The model under review builds one solid part; all positions refer to its coordinate system, in mm. Face numbers are marked on the shaded views. Round coordinates to 2 decimals unless told otherwise and drop trailing zeros. Loops run counter-clockwise (first coordinate to the right, second up) from the corner with the lowest first, then second, coordinate; pieces in that order, holes last. Notation, with made-up numbers: M 16,48.5 L 24,48.5 A18 cw 24,62.5 Z; hole C -21,-4 d4. An arc over 180 degrees is marked long. Answer in a Markdown table with one row per item. Add a question column.
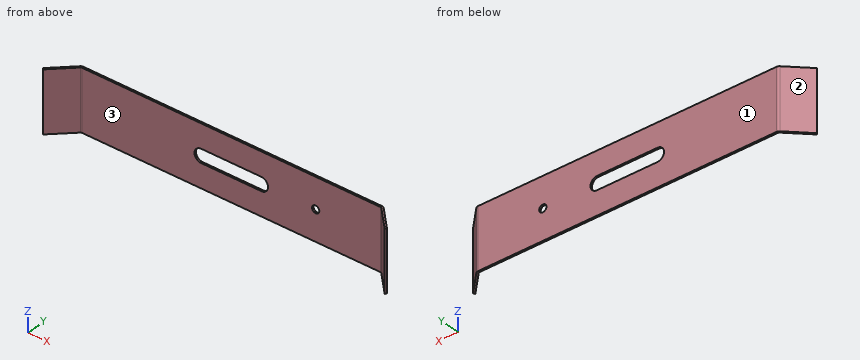
Autodesk Inventor part; units mm, degrees
ref_plane "YZ Plane" through (0, 0, 0) normal (1, 0, 0) x (0, 1, 0)
ref_plane "XZ Plane" through (0, 0, 0) normal (0, 1, 0) x (-1, 0, 0)
ref_plane "XY Plane" through (0, 0, 0) normal (0, 0, 1) x (1, 0, 0)
sketch "Sketch4" plane through (0, 0, 0) normal (0, 1, 0) x (-1, 0, 0)
  line L0 (125, 25) -> (-125, 25)
  line L1 (-125, 25) -> (-125, -25)
  line L2 (-125, -25) -> (125, -25)
  line L3 (125, -25) -> (125, 25)
  line L4 (125, 25) -> (-125, -25) construction
  line L5 (-125, 25) -> (125, -25) construction
  line L6 (25, 0) -> (-25, 0) construction
  line L7 (25, 5.5) -> (-25, 5.5)
  line L8 (-25, -5.5) -> (25, -5.5)
  arc A0 (25, -5.5) -> (25, 5.5) centre (25, 0) ccw
  arc A1 (-25, 5.5) -> (-25, -5.5) centre (-25, 0) ccw
  point P0 (0, 0)
  point P1 (0, 0)
  dimension "d17" = 250
  dimension "d18" = 50
  dimension "d19" = 50
  dimension "d20" = 11
extrude "Plate3" add sketch "Sketch4" along normal blind 1.5
sketch "Sketch6" plane through (-123.9393, 0.4393, -25) normal (-0.7071068, 0.7071068, 0) x (-0.7071068, -0.7071068, 0)
  line L0 (0, 50) -> (0, 0)
  line L1 (0, 0) -> (25, 0)
  line L2 (25, 0) -> (25, 50)
  line L3 (25, 50) -> (0, 50)
edge flange "Flange3" height 25 angle 45 thickness 1.5 bend radius 1.5 thickness toward (-0.7071068, 0.7071068, 0) relief tear relief width 1.5 relief depth 0.75 corner gap 1.5 corner form 0 edges at (-125, 0, 0) (125, 0, 0) wall of the first edge with corners at (-123.9393, 0.4393, 25) (-123.9393, 0.4393, -25) (-141.617, -17.2383, -25) (-141.617, -17.2383, 25)
bend "Bend3"
corner "Corner3"
sketch "Sketch7" plane through (0, 1.5, 0) normal (0, 1, 0) x (1, 0, 0)
  circle A0 centre (70, 0) radius 3
  point P0 (0, 0)
  dimension "d43" = 70
  dimension "d44" = 6
extrude "Cut2" cut sketch "Sketch7" against normal blind 1.5
equation "\"d41\" = Thickness"
equation "\"d2\" = Thickness"
equation "\"d31\" = BendReliefWidth"
equation "\"d32\" = BendReliefDepth"
equation "\"d33\" = MinimumRemnant"
equation "\"d34\" = TransitionRadius"
equation "\"d37\" = BendRadius"
equation "\"d38\" = CornerReliefSize"
equation "\"d39\" = GapSize"
equation "\"d40\" = JacobiRadiusSize"
equation "\"BendRadius\" = Thickness"
equation "\"BendReliefWidth\" = Thickness"
equation "\"BendReliefDepth\" = 0.5 * Thickness"
equation "\"CornerReliefSize\" = 4 * Thickness"
equation "\"MinimumRemnant\" = 2 * Thickness"
equation "\"TransitionRadius\" = BendRadius"
equation "\"JacobiRadiusSize\" = BendRadius"
equation "\"GapSize\" = Thickness"
properties part number "2309HCMUTE-CDT23_TAY-GAT" material "Stainless Steel"
1. For pin 1 Ø10 at (y, z) = (-2, 10.5) entering from -X; pin 2 Ø1 at (y, z) = (-10.5, 13) entering from -X; pin 3 Ø25 at (x, z) = (-12.5, -2.5) entering from -Y, all flat-tipped, find the tip position at first contact; note any pin that passes through.
2. Mouldability with a two-part tool opening along X and no side actions: class the marked faces 1, 2 and 3 as released by +X, released by -X, zero draft, split by the parting line, or undercut.
3. Take a section at D-D, the plane x = 41. State the section outline as (y, z) points.
4. To check wall thickness, follow probe 1 along X at (y, z) = (0.8, 0); probe 2 along X at (y, z) = (0.6, 0); probe 3 along Z at (x, y) = (70, 0.3). State the ranges of each line that lie inside material, in increasing order.
5. Take a section at C-C, the plane z = -10.5. State the section outline as (x, y) points.
6. Take a section at A-A, the plane x = 70. State the section outline as (y, z) points, and give its area (3 significant figures).
7. Take a section at B-B, the plane y = -7. State the section outline as (x, z) points, and give its area (3 significant figures).
Check sheet entries:
| question | item | result |
|---|---|---|
| 1 | pin 1 | stops at x = -133.5 |
| 1 | pin 2 | stops at x = -137.5 |
| 1 | pin 3 | stops at y = 0 |
| 2 | face 1 | zero draft |
| 2 | face 2 | released by -X |
| 2 | face 3 | undercut |
| 3 | outline | M 0,-25 L 1.5,-25 L 1.5,25 L 0,25 Z |
| 4 | probe 1 | x = -125.68 to -30.5, 30.5 to 67, 73 to 125.68 |
| 4 | probe 2 | x = -125.9 to -30.5, 30.5 to 67, 73 to 125.9 |
| 4 | probe 3 | z = -25 to -3, 3 to 25 |
| 5 | outline | M -142.68,-16.18 L -141.62,-17.24 L -124.82,-0.44 A1.5 cw -123.76,0 L 123.76,0 A1.5 cw 124.82,-0.44 L 141.62,-17.24 L 142.68,-16.18 L 125.88,0.62 A3 ccw 123.76,1.5 L -123.76,1.5 A3 ccw -125.88,0.62 Z |
| 6 | outline | M 0,-25 L 1.5,-25 L 1.5,-3 L 0,-3 Z; M 0,3 L 1.5,3 L 1.5,25 L 0,25 Z |
| 6 | area | 66.0 mm^2 |
| 7 | outline | M -133.5,-25 L -131.38,-25 L -131.38,25 L -133.5,25 Z; M 131.38,-25 L 133.5,-25 L 133.5,25 L 131.38,25 Z |
| 7 | area | 212 mm^2 |
